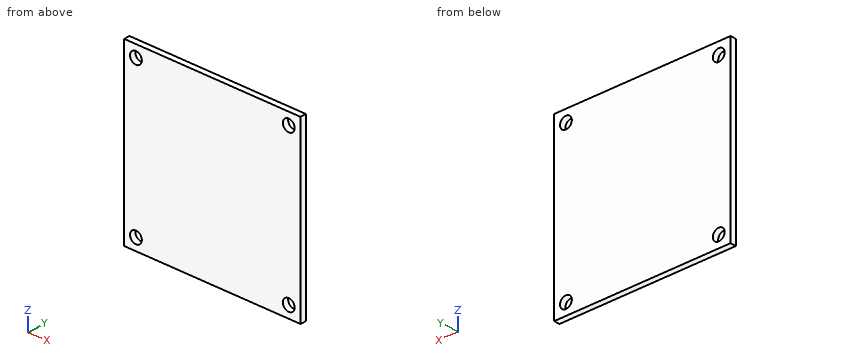
Autodesk Inventor part; units mm, degrees
ref_plane "YZ Plane" through (0, 0, 0) normal (1, 0, 0) x (0, 1, 0)
ref_plane "XZ Plane" through (0, 0, 0) normal (0, 1, 0) x (-1, 0, 0)
ref_plane "XY Plane" through (0, 0, 0) normal (0, 0, 1) x (1, 0, 0)
sketch "Sketch1" plane through (0, 0, 0) normal (0, 1, 0) x (-1, 0, 0)
  line L0 (0, 0) -> (381, 0)
  line L1 (381, 0) -> (381, -381)
  line L2 (381, -381) -> (0, -381)
  line L3 (0, -381) -> (0, 0)
extrude "Extrusion1" add sketch "Sketch1" along normal blind 12.7
sketch "Sketch2" plane through (0, 12.7, 0) normal (0, 1, 0) x (1, 0, 0)
  circle A0 centre (-25.4, 25.4) radius 12.7
  line L0 (0, 0) -> (0, 381)
  line L1 (-381, 0) -> (0, 0)
extrude "Extrusion2" cut sketch "Sketch2" against normal blind 12.7
sketch "Sketch3" plane through (0, 12.7, 0) normal (0, 1, 0) x (1, 0, 0)
  circle A0 centre (-25.4, 355.6) radius 12.7
  line L0 (0, 381) -> (-381, 381)
  line L1 (0, 0) -> (0, 381)
extrude "Extrusion3" cut sketch "Sketch3" against normal blind 12.7
sketch "Sketch4" plane through (0, 12.7, 0) normal (0, 1, 0) x (1, 0, 0)
  circle A0 centre (-355.6, 25.4) radius 12.7
  line L0 (-381, 381) -> (-381, 0)
  line L1 (-381, 0) -> (0, 0)
extrude "Extrusion4" cut sketch "Sketch4" against normal blind 12.7
sketch "Sketch5" plane through (0, 12.7, 0) normal (0, 1, 0) x (1, 0, 0)
  circle A0 centre (-355.6, 355.6) radius 12.7
  line L0 (0, 381) -> (-381, 381)
  line L1 (-381, 381) -> (-381, 0)
  point P0 (0, 0)
extrude "Extrusion5" cut sketch "Sketch5" against normal blind 12.7
properties part number "upside"
The listing builds one solid part. Answer for the finished solid, in the listing's coordinates (mm). Coordinates: 2 decimals unless noted, no trailing zeros. Loops run counter-clockwise (first coordinate to the right, second up) from the corner with the lowest first, then second, coordinate; pieces in that order, holes last. Notation, with made-up numbers: (76, 74.5) -> (90, 74.5) arc R24 cw to (90, 107.5) -> close; hole circle Ø7 at (84.5, 80.25). An arc over 180 degrees is marked (long way). Write item = value, one per line. Start each with the question number.
1) Straight lines are drawn through the part: line 1 (X direction, y = 7.5, z = -355.6); line 2 (Z direction, x = -362, y = 8.75). For each, find the intervals that lie inside material, in ascending order. Write a range as from..to.
2) A cutting plane is placed at A-A (x = -355.6). Give the vertices of the cut face in (y, z), then the cut area to 3 significant figures.
3) A cutting plane is placed at B-B (z = -25.4). Give the vertices of the cut face in (x, y).
4) Given pin 1 Ø20.5 at (x, z) = (-25.4, -25.4) entering from -Y, flat-ended and moving along its own axis, determine where the tip first touches the part or whether it passes through.
Responses:
q1.line_1 = -381..-368.3, -342.9..-38.1, -12.7..0
q1.line_2 = -381..-366.57, -344.63..-36.37, -14.43..0
q2.outline = (0, -381) -> (12.7, -381) -> (12.7, -368.3) -> (0, -368.3) -> close; (0, -342.9) -> (12.7, -342.9) -> (12.7, -38.1) -> (0, -38.1) -> close; (0, -12.7) -> (12.7, -12.7) -> (12.7, 0) -> (0, 0) -> close
q2.area = 4,190 mm²
q3.outline = (-381, 0) -> (-368.3, 0) -> (-368.3, 12.7) -> (-381, 12.7) -> close; (-342.9, 0) -> (-38.1, 0) -> (-38.1, 12.7) -> (-342.9, 12.7) -> close; (-12.7, 0) -> (0, 0) -> (0, 12.7) -> (-12.7, 12.7) -> close
q4.pin_1 = through
